CAD build for the part. Positions are in the model's coordinates, mm. Face numbers are marked on the shaded views. Round coordinates to 2 decimals unless told otherwise and drop trailing zeros. Order: outer loops, then holes, each group sorted by start corner. A loop starts at its lowest first (then second) coordinate and runs counter-clockwise, first axis right, second up. Notation, with made-up numbers: M 11,81.25 L 31,81.25 A29 cw 31,102.25 Z; hole C 14,31 d8. An arc over 180 degrees is marked long. Put each result on its own line as item: value.
```python
from build123d import *

# Parameters (mm, degrees)
BOSS_EXTRUDE1_DEPTH = 6
BOSS_EXTRUDE2_DEPTH = 90
BOSS_EXTRUDE3_DEPTH = 3
FILLET1_R           = 3
FILLET2_R           = 3
FILLET3_R           = 30
SKETCH4_W           = 4
SKETCH4_H           = 2
CUT_EXTRUDE1_DEPTH  = 136.546495779
CUT_EXTRUDE2_DEPTH  = 175.004604959


with BuildPart() as part:
    # Sketch2 → Boss-Extrude1 (new body)
    with BuildSketch(Plane.XY):
        Polygon((2.5, 4.05), (0, 4.05), (0, -4.05), (10.5, -4.05), (10.5, 30.95), (2.5, 30.95), align=None)
        Polygon((-2.04, 7.95), (0, 7.95), (0, -7.95), (-2.04, -7.95), (-6.152414984, -4.048), (-6.152414984, 4.048), align=None)
    extrude(amount=BOSS_EXTRUDE1_DEPTH)

    # Sketch2<3> → Boss-Extrude2 (add)
    with BuildSketch(Plane.XY):
        Polygon((-49.5, 30.95), (92.5, 30.95), (92.5, -19.05), (95.5, -19.05), (95.5, 33.95), (-49.5, 33.95), align=None)
    extrude(amount=BOSS_EXTRUDE2_DEPTH)

    # Sketch2<4> → Boss-Extrude3 (add)
    with BuildSketch(Plane.XY):
        Polygon((10.5, 30.95), (10.5, -4.05), (10.5, -19.05), (92.5, -19.05), (92.5, 30.95), (30.5, 30.95), align=None)
    extrude(amount=BOSS_EXTRUDE3_DEPTH)

    # Fillet1
    fillet1_edges = [part.edges().sort_by_distance(p)[0] for p in [
        (10.5, 13.45, 3),
    ]]
    fillet(fillet1_edges, radius=FILLET1_R - 0.0001)  # a hair under: the kernel refuses the full size

    # Fillet2
    fillet2_edges = [part.edges().sort_by_distance(p)[0] for p in [
        (10.5, 13.45, 6),
    ]]
    fillet(fillet2_edges, radius=FILLET2_R)

    # Fillet3
    fillet3_edges = [part.edges().sort_by_distance(p)[0] for p in [
        (-49.5, 32.45, 90),
    ]]
    fillet(fillet3_edges, radius=FILLET3_R)

    # Sketch4 → Cut-Extrude1 (cut, through all)
    with BuildSketch(Plane(origin=(0, 0, 0), x_dir=(-1, 0, 0), z_dir=(0, 0, -1))):
        with Locations((4.152414984, 0)):
            Rectangle(SKETCH4_W, SKETCH4_H)
    extrude(amount=-CUT_EXTRUDE1_DEPTH, mode=Mode.SUBTRACT)

    # Sketch5 → Cut-Extrude2 (cut, through all)
    with BuildSketch(Plane(origin=(95.5, 0, 0), x_dir=(0, 0, -1), z_dir=(1, 0, 0))):
        Polygon((-8.799025007, -19.05), (-90, 1.95), (-90, -19.05), align=None)
    extrude(amount=-CUT_EXTRUDE2_DEPTH, mode=Mode.SUBTRACT)


solid = part.part
```
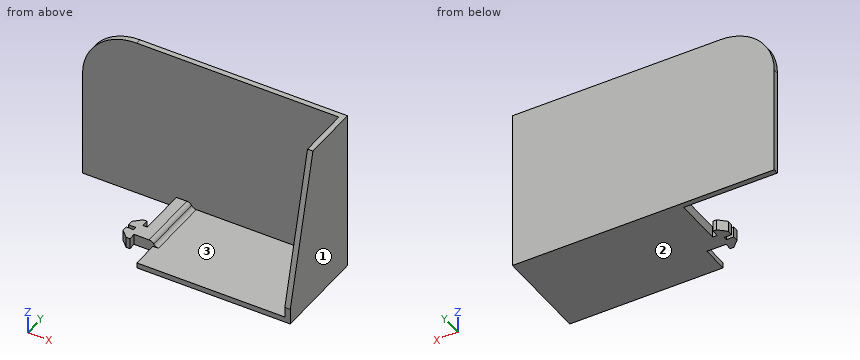
Item 1: Mould opens along X. For the marked faces 1, 2 and 3 say: pulls with the +X half, pulls with the -X half, needs draft (parallel to the pull), parting line crosses it, or undercut.
Answers below:
face 1: pulls with the +X half
face 2: needs draft
face 3: undercut
Item 2: Band-saw the part on B-B on x = 28.5. Give the cut face in (y, z), and give its area (3 significant figures).
Answers below:
outline: M -19.05,0 L 33.95,0 L 33.95,90 L 30.95,90 L 30.95,3 L -19.05,3 Z
area: 420 mm²
Item 3: Band-saw the part on C-C on z = 76. Give the cut face in (x, y).
Answers below:
outline: M -44.88,30.95 L 92.5,30.95 L 92.5,-1.67 L 95.5,-1.67 L 95.5,33.95 L -44.88,33.95 Z
Item 4: Probe line 1 along X through (y, z) = (23.5, 42.5); line 2 along Y through (x, z) = (55.5, 18.5); line 3 along Z through (x, y) = (72.5, 16.5). List the from-to ranges inside material, lowest first. Write a range as [from, to].
Answers below:
line 1: [92.5, 95.5]
line 2: [30.95, 33.95]
line 3: [0, 3]
Item 5: Pin check, flat tips, straight feed: P1, Ø4, axis at x = 28.5, y = 9, coming from the +Z side; P2, Ø1.5, axis at x = -31, z = 45, coming from the -Y side; P3, Ø1.8, axis at x = 4, z = 3.5, coming from the -Y side. Stop position of each tip, or through.
Answers below:
P1: z = 3
P2: y = 30.95
P3: y = -4.05
Item 6: Band-saw the part on D-D on x = -30. Give the cut face in (y, z), and give its area (3 significant figures).
Answers below:
outline: M 30.95,0 L 33.95,0 L 33.95,88.1 L 30.95,88.1 Z
area: 264 mm²
Item 7: Band-saw the part on A-A on x = -4. Give the cut face in (y, z), and give its area (3 significant figures).
Answers below:
outline: M -6.09,0 L -1,0 L -1,6 L -6.09,6 Z; M 1,0 L 6.09,0 L 6.09,6 L 1,6 Z; M 30.95,0 L 33.95,0 L 33.95,90 L 30.95,90 Z
area: 331 mm²
